The listing builds one solid part. Answer for the finished solid, in the listing's coordinates (mm). A direction names the side the tool comes from. Round coordinates to 2 decimals unless told otherwise and drop trailing zeros. Order: outer loops, then holes, each group sorted by start corner. A loop starts at its lowest first (then second) coordinate and runs counter-clockwise, first axis right, second up. Notation, with made-up numbers: (48, 24.5) - (73, 24.5) arc R5 cw to (73, 33.5) - close; hole circle Ø2 at (-33.75, 70). An arc over 180 degrees is marked (long way). One line per item, written item: value. Start each with the question number.
1. Straight lines are drawn through the part: line 1 (X direction, y = 2.5, z = 12.5); line 2 (Y direction, x = 20, z = 9.5); line 3 (Z direction, x = 17, y = 1.35). For each, find the intervals that lie inside material, in ascending order.
2. Section C-C, the plane z = 0 is taken. Give the vertices of the cut face in (x, y).
3. Flat-ended cylindrical pins translate along their axes: P1, Ø4, axis at x = -18, z = -7, coming from the -Y side; P2, Ø3, axis at y = 1.5, z = 12.5, coming from the +X side; P3, Ø3.5, axis at x = -21.65, z = 12.5, coming from the +Y side. Find the tip coordinate at first contact, or state that the pin passes through.
4. A tool of negligible diameter and unlimited length cuts with its end or side. For faces 1 (the flat face through (-22, 0.7, 13)), 2 (the flat face through (18, 3, 8)), 3 (the cylindrical face through (0.1, -1, -22.1)), from which of +Z, -Z, +X, -X, +Y, -Y can it reach the whole face along a straight path? Write none if from no direction.
5. Section B-B, the plane z = -6 is taken. Give the vertices of the cut face in (x, y).
6. For a pull along X with two mould halves and no side action, classify faces 4 (the flat face through (-22, -2, 13)), 5 (the cylindrical face through (-10.94, 1.48, -20.59)), 6 (the cylindrical face through (-23.42, -0.99, 14.8)), 7 (the cylindrical face through (12.476, 1.479, 19.776)) as released by +X, released by -X, zero draft, split by the parting line, or undercut.
7. Section A-A, the plane x = 0 is taken. Give the vertices of the cut face in (y, z), then the cut area to 3 significant figures.
8. Section D-D, the plane y = 2 is taken. Count the separate pieces of the cut face and the enclosed holes in it, then the cut area to 3 significant figures.
from build123d import *

# Parameters (mm, degrees)
SKETCH1_R                = 19
BOSS_EXTRUDE1_DEPTH      = 3.5
SKETCH2_R                = 30
SKETCH2_R_2              = 19
SKETCH2_R_3              = 2.8
BOSS_EXTRUDE2_DEPTH      = 3
BOSS_EXTRUDE3_DEPTH      = 2
BOSS_EXTRUDE3_DEPTH_BACK = 3
SKETCH4_R                = 2.9
SKETCH5_R                = 5
BOSS_EXTRUDE4_DEPTH      = 3
CUT_EXTRUDE1_START       = -10
SKETCH3_R                = 19
CUT_EXTRUDE1_DEPTH       = 10
SKETCH6_R                = 3.2
SKETCH6_R_2              = 2.9
CUT_EXTRUDE2_DEPTH       = 2.3
CUT_EXTRUDE3_START       = -13
CUT_EXTRUDE3_DEPTH       = 13
FILLET1_R                = 10
FILLET2_R                = 5


with BuildPart() as part:
    # Sketch1 → Boss-Extrude1 (new body)
    with BuildSketch(Plane(origin=(0, 0, 0), x_dir=(1, 0, 0), z_dir=(0, 1, 0))):
        with Locations(Location((0, 0, 0), (0, 0, 270))):
            Circle(SKETCH1_R)
    extrude(amount=BOSS_EXTRUDE1_DEPTH)

    # Sketch2 → Boss-Extrude2 (add)
    with BuildSketch(Plane(origin=(0, 0, 0), x_dir=(1, 0, 0), z_dir=(0, 1, 0))):
        with Locations(Location((0, 0, 0), (0, 0, 270))):
            Circle(SKETCH2_R)
        with Locations(Location((0, 0, 0), (0, 0, 270))):
            Circle(SKETCH2_R_2, mode=Mode.SUBTRACT)
        with Locations(Location((0, 25, 0), (0, 0, 270))):
            Circle(SKETCH2_R_3, mode=Mode.SUBTRACT)
        with Locations(Location((21.650635095, -12.5, 0), (0, 0, 270))):
            Circle(SKETCH2_R_3, mode=Mode.SUBTRACT)
        with Locations(Location((-21.650635095, -12.5, 0), (0, 0, 270))):
            Circle(SKETCH2_R_3, mode=Mode.SUBTRACT)
    extrude(amount=BOSS_EXTRUDE2_DEPTH)

    # Sketch4 → Boss-Extrude3 (add, two sides: drawn at the far end of the back side and taken through both)
    with BuildSketch(Plane.XZ.offset(-BOSS_EXTRUDE3_DEPTH_BACK)):
        with Locations(Location((-21.650635095, 12.5, 0), (0, 0, 270))):
            Circle(SKETCH4_R)
        with Locations(Location((21.650635095, 12.5, 0), (0, 0, 270))):
            Circle(SKETCH4_R)
        with Locations(Location((0, -25, 0), (0, 0, 270))):
            Circle(SKETCH4_R)
    extrude(amount=BOSS_EXTRUDE3_DEPTH + BOSS_EXTRUDE3_DEPTH_BACK)

    # Sketch5 → Boss-Extrude4 (add)
    with BuildSketch(Plane(origin=(0, 3, 0), x_dir=(1, 0, 0), z_dir=(0, 1, 0))):
        with Locations((-26.103110985, -14.7860609)):
            Circle(SKETCH5_R)
        with Locations((0.246451131, 29.99898768)):
            Circle(SKETCH5_R)
        with Locations((25.856659853, -15.212926781)):
            Circle(SKETCH5_R)
    extrude(amount=-BOSS_EXTRUDE4_DEPTH)

    # Sketch3 → Cut-Extrude1 (cut)
    with BuildSketch(Plane(origin=(0, 3.5, 0), x_dir=(1, 0, 0), z_dir=(0, 1, 0)).offset(CUT_EXTRUDE1_START)):
        with Locations(Location((0, 0, 0), (0, 0, 270))):
            Circle(SKETCH3_R)
    extrude(amount=CUT_EXTRUDE1_DEPTH, mode=Mode.SUBTRACT)

    # Sketch6 → Cut-Extrude2 (cut)
    with BuildSketch(Plane(origin=(0, 3, 0), x_dir=(1, 0, 0), z_dir=(0, 1, 0))):
        with Locations(Location((0, 25, 0), (0, 0, 270))):
            Circle(SKETCH6_R)
        with Locations(Location((21.650635095, -12.5, 0), (0, 0, 90))):
            Circle(SKETCH6_R_2)
        with Locations(Location((-21.650635095, -12.5, 0), (0, 0, 90))):
            Circle(SKETCH6_R_2)
    extrude(amount=-CUT_EXTRUDE2_DEPTH, mode=Mode.SUBTRACT)

    # Sketch7 → Cut-Extrude3 (cut)
    with BuildSketch(Plane(origin=(0, 3, 0), x_dir=(1, 0, 0), z_dir=(0, 1, 0)).offset(CUT_EXTRUDE3_START)):
        with BuildLine():
            ThreePointArc((-29.54423259, -5.20944533), (-25.980762114, 15), (-10.2606043, 28.190778624))
            Line((-10.2606043, 28.190778624), (-13.773984089, 37.84371026))
            Line((-13.773984089, 37.84371026), (-43.939319858, -7.747687605))
            Line((-43.939319858, -7.747687605), (-29.54423259, -5.20944533))
        make_face()
        with BuildLine():
            ThreePointArc((-21.729408673, -3.831481024), (-19.108521295, 11.032309914), (-7.546544436, 20.733960432))
            Line((-7.546544436, 20.733960432), (-10.2606043, 28.190778624))
            ThreePointArc((-10.2606043, 28.190778624), (-25.980762114, 15), (-29.54423259, -5.20944533))
            Line((-29.54423259, -5.20944533), (-21.729408673, -3.831481024))
        make_face()
        with BuildLine():
            Line((15.259965643, 41.926411025), (10.2606043, 28.190778624))
            ThreePointArc((10.2606043, 28.190778624), (25.980762114, 15), (29.54423259, -5.20944533))
            Line((29.54423259, -5.20944533), (39.660606503, -6.993234998))
            Line((39.660606503, -6.993234998), (15.259965643, 41.926411025))
        make_face()
        with BuildLine():
            Line((10.2606043, 28.190778624), (7.546544436, 20.733960432))
            ThreePointArc((7.546544436, 20.733960432), (18.074278438, 12.65574601), (22.064619828, 0))
            ThreePointArc((22.064619828, 0), (21.980657288, -1.92305833), (21.729408673, -3.831481024))
            Line((21.729408673, -3.831481024), (29.54423259, -5.20944533))
            ThreePointArc((29.54423259, -5.20944533), (25.980762114, 15), (10.2606043, 28.190778624))
        make_face()
        with BuildLine():
            Line((28.679354216, -34.17872342), (19.283628291, -22.981333294))
            ThreePointArc((19.283628291, -22.981333294), (0, -30), (-19.283628291, -22.981333294))
            Line((-19.283628291, -22.981333294), (-25.886622414, -30.850475262))
            Line((-25.886622414, -30.850475262), (28.679354216, -34.17872342))
        make_face()
        with BuildLine():
            Line((19.283628291, -22.981333294), (14.182864238, -16.902479408))
            ThreePointArc((14.182864238, -16.902479408), (0, -22.064619828), (-14.182864238, -16.902479408))
            Line((-14.182864238, -16.902479408), (-19.283628291, -22.981333294))
            ThreePointArc((-19.283628291, -22.981333294), (0, -30), (19.283628291, -22.981333294))
        make_face()
    extrude(amount=CUT_EXTRUDE3_DEPTH, mode=Mode.SUBTRACT)

    # Fillet1
    # the kernel refuses this fillet: 10 mm, written as the material it adds along each edge
    with BuildSketch(Plane(origin=(-21.729408673, 0, 3.831481024), x_dir=(-0.9848077530122133, 0, 0.17364817766690055), z_dir=(0, 1, 0)), Plane(origin=(14.182864238, 0, 16.902479408), x_dir=(0.6427876096865253, 0, 0.7660444431189899), z_dir=(0, 1, 0)), Plane(origin=(7.546544436, 0, -20.733960432), x_dir=(0.34202014332569675, 0, -0.9396926207858982), z_dir=(0, 1, 0))) as fillet1_piece_1:
        with BuildLine():
            CenterArc((8.404377584, -9.988996017), FILLET1_R, 92.688143309, 69.160575724)
            Line((-1.097995304, -6.873725644), (-1.288042762, -6.811420237))
            ThreePointArc((-1.288042762, -6.811420237), (-0.473724072, -3.448886874), (-0.2, 0))
            Line((-0.2, 0), (0, 0.2))
            ThreePointArc((0, 0.2), (3.967690086, 0.2), (7.926000224, 0.19977992))
            Line((7.926000224, 0.19977992), (7.935380172, 0))
        make_face()
    extrude(amount=3)
    with BuildSketch(Plane(origin=(-14.182864238, 0, 16.902479408), x_dir=(0.8578464941811706, 0, 0.5139060151633514), z_dir=(0, 1, 0)), Plane(origin=(21.729408673, 0, 3.831481024), x_dir=(0.01613241719851076, 0, -0.9998698640899891), z_dir=(0, 1, 0)), Plane(origin=(-7.546544436, 0, -20.733960432), x_dir=(-0.8739789113796794, 0, 0.48596384892663586), z_dir=(0, 1, 0))) as fillet1_piece_2:
        with BuildLine():
            CenterArc((8.538251552, -9.87480959), FILLET1_R, 99.075640483, 69.160575724)
            Line((-1.251712984, -7.836036823), (-1.447512274, -7.795261367))
            ThreePointArc((-1.447512274, -7.795261367), (-0.823352684, -3.886470761), (-0.197496192, 0.03154765))
            Line((-0.197496192, 0.03154765), (0.03154765, 0.197496192))
            ThreePointArc((0.03154765, 0.197496192), (3.480434524, -0.07622788), (6.929321399, 0.197496192))
            Line((6.929321399, 0.197496192), (6.960869049, 0))
        make_face()
    extrude(amount=3)

    # Fillet2
    fillet2_edges = [part.edges().sort_by_distance(p)[0] for p in [
        (-19.283628291, 1.5, 22.981333294),
        (19.283628291, 1.5, 22.981333294),
        (29.54423259, 1.5, 5.20944533),
        (10.2606043, 1.5, -28.190778624),
        (-10.2606043, 1.5, -28.190778624),
        (-29.54423259, 1.5, 5.20944533),
    ]]
    fillet(fillet2_edges, radius=FILLET2_R)


solid = part.part
Answer list:
1. line 1: x = -30.55 to -24.55, -18.75 to -14.31, 14.31 to 18.75, 24.55 to 30.06
1. line 2: y = 0 to 3
1. line 3: z = -14.07 to -8.49, 8.49 to 21.09
2. outline: (-22.83, 0) - (-19, 0) - (-19, 3) - (-22.83, 3) - close; (19, 0) - (22.83, 0) - (22.83, 3) - (19, 3) - close
3. P1: stops at y = 0
3. P2: stops at x = 30.71
3. P3: stops at y = 0.7
4. face 1: +Y
4. face 2: +Z, -Z, +X, -X, +Y
4. face 3: -Y
5. outline: (-21.23, 0) - (-18.03, 0) - (-18.03, 3) - (-21.23, 3) - close; (18.03, 0) - (21.23, 0) - (21.23, 3) - (18.03, 3) - close
6. face 4: zero draft
6. face 5: released by -X
6. face 6: undercut
6. face 7: undercut
7. outline: (-2, -27.9) - (0, -27.9) - (0, -34.99) - (3, -34.99) - (3, -28.2) - (0.7, -28.2) - (0.7, -21.8) - (3, -21.8) - (3, -19) - (0, -19) - (0, -22.1) - (-2, -22.1) - close; (0, 19) - (3, 19) - (3, 22.06) - (0, 22.06) - close
7. area: 54.1 mm²
8. separate pieces: 1
8. enclosed holes: 4
8. area: 919 mm²
